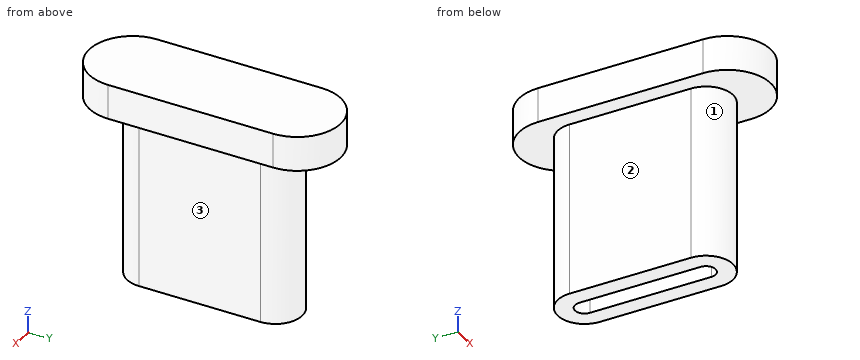
```python
from build123d import *

# Parameters (mm, degrees)
BOSS_EXTRU_3_DEPTH = 10
BOSS_EXTRU_4_DEPTH = 2


with BuildPart() as part:
    # Esquisse1 → Boss.-Extru.3 (new body)
    with BuildSketch(Plane.XY):
        with BuildLine():
            Line((-1.517140129, 11.017733261), (-1.517140129, 4.017733261))
            ThreePointArc((-1.517140129, 4.017733261), (0.032859871, 2.467733261), (1.582859871, 4.017733261))
            Line((1.582859871, 4.017733261), (1.582859871, 11.017733261))
            ThreePointArc((1.582859871, 11.017733261), (0.032859871, 12.567733261), (-1.517140129, 11.017733261))
        make_face()
        with BuildLine():
            Line((-0.517140129, 11.017733261), (-0.517140129, 4.017733261))
            ThreePointArc((-0.517140129, 4.017733261), (0.032859871, 3.467733261), (0.582859871, 4.017733261))
            Line((0.582859871, 4.017733261), (0.582859871, 11.017733261))
            ThreePointArc((0.582859871, 11.017733261), (0.032859871, 11.567733261), (-0.517140129, 11.017733261))
        make_face(mode=Mode.SUBTRACT)
    extrude(amount=-BOSS_EXTRU_3_DEPTH)

    # Esquisse3 → Boss.-Extru.4 (add)
    with BuildSketch(Plane.XY):
        with BuildLine():
            Line((-2.5, 2.767733261), (-2.5, 12.267733261))
            ThreePointArc((-2.5, 12.267733261), (0, 14.767733261), (2.5, 12.267733261))
            Line((2.5, 12.267733261), (2.5, 2.767733261))
            ThreePointArc((2.5, 2.767733261), (0, 0.267733261), (-2.5, 2.767733261))
        make_face()
    extrude(amount=BOSS_EXTRU_4_DEPTH)


solid = part.part
```
Model file for the job. Use its own axes, mm. Face numbers are marked on the shaded views. A direction names the side the tool comes from. Coordinates: 2 decimals unless noted, no trailing zeros. Loops run counter-clockwise (first coordinate to the right, second up) from the corner with the lowest first, then second, coordinate; pieces in that order, holes last. Notation, with made-up numbers: (-15, 66.25) - (-7, 66.25) arc R6 ccw to (-7, 73.25) - close; hole circle Ø4 at (82, 59). An arc over 180 degrees is marked (long way). Answer as a JSON object with one key per item and string values. Group by question number.
(1) Cut at B-B (y = 5). Give the cut face in (x, z), then the cut area to 3 significant figures.
(2) Tool access for the marked faces 1, 2 and 3: list every direction of +Z, -Z, +X, -X, +Y, -Y with a clear straight run to the whole face (end or side of a thin tool).
(3) Probe line 1 along X through (y, z) = (4, -2); line 2 along Y through (x, z) = (-0.3, -0.75); line 3 along Z through (x, y) = (1.95, 1.75). List the from-to ranges inside material, lowest first.
(4) Cut at D-D (x = 0). Give the cut face in (y, z).
(5) Flat gauge pins, fed straight in: pin 1 (3 mm diameter, centred on x = -1, z = -3, fed in from -Y); pin 2 (2 mm diameter, centred on y = 7.5, z = -6, fed in from +X); pin 3 (5 mm diameter, centred on y = 9.5, z = -8.5, fed in from -X). Where does each tip first touch, or does it go through?
(6) Cut at A-A (z = -4.5). Give the cut face in (x, y), then the cut area to 3 significant figures.
(7) Cut at C-C (x = -0.85). Give the cut face in (y, z), then the cut area to 3 significant figures.
Geometry says:
{
 "1": {"outline": "(-2.5, 0) - (-1.52, 0) - (-1.52, -10) - (-0.52, -10) - (-0.52, 0) - (0.58, 0) - (0.58, -10) - (1.58, -10) - (1.58, 0) - (2.5, 0) - (2.5, 2) - (-2.5, 2) - close", "area": "30.0 mm^2"},
 "2": {"face 1": "-Z, -Y", "face 2": "-Z, -X, +Y, -Y", "face 3": "-Z, +X, +Y, -Y"},
 "3": {"line 1": "x = -1.52 to -0.52, 0.58 to 1.58", "line 2": "y = 2.5 to 3.58, 11.46 to 12.53", "line 3": "z = 0 to 2"},
 "4": {"outline": "(0.27, 0) - (2.47, 0) - (2.47, -10) - (3.47, -10) - (3.47, 0) - (11.57, 0) - (11.57, -10) - (12.57, -10) - (12.57, 0) - (14.77, 0) - (14.77, 2) - (0.27, 2) - close"},
 "5": {"pin 1": "stops at y = 2.47", "pin 2": "stops at x = 1.58", "pin 3": "stops at x = -1.52"},
 "6": {"outline": "(-1.52, 4.02) arc R1.55 ccw to (1.58, 4.02) - (1.58, 11.02) arc R1.55 ccw to (-1.52, 11.02) - close; hole (-0.52, 4.02) arc R0.55 ccw to (0.58, 4.02) - (0.58, 11.02) arc R0.55 ccw to (-0.52, 11.02) - close", "area": "20.6 mm^2"},
 "7": {"outline": "(0.42, 0) - (2.74, 0) - (2.74, -10) - (12.29, -10) - (12.29, 0) - (14.62, 0) - (14.62, 2) - (0.42, 2) - close", "area": "124 mm^2"}
}
